```python
from build123d import *

# Parameters (mm, degrees)
BOSS_EXTRUDE1_DEPTH = 1.5875
CUT_EXTRUDE1_DEPTH  = 288.311537501
CUT_EXTRUDE2_DEPTH  = 1.5875
FILLET1_R           = 2.54


with BuildPart() as part:
    # Sketch2 → Boss-Extrude1 (new body)
    with BuildSketch(Plane(origin=(0, 0, 0), x_dir=(1, 0, 0), z_dir=(0, 1, 0))):
        Polygon((-122.047, 0), (0, 0), (122.047, 0), (11.684, -253.746), (6.35, -253.746), (6.35, -260.096), (-6.35, -260.096), (-6.35, -253.746), (-11.684, -253.746), align=None)
    extrude(amount=BOSS_EXTRUDE1_DEPTH)

    # Sketch3 → Cut-Extrude1 (cut, through all)
    with BuildSketch(Plane(origin=(0, 1.5875, 0), x_dir=(1, 0, 0), z_dir=(0, 1, 0))):
        Polygon((41.529, 0), (41.529, -4.7625), (119.975622372, -4.7625), (122.047, 0), align=None)
        Polygon((-119.975622372, -4.7625), (-122.047, 0), (-41.529, 0), (-41.529, -4.7625), align=None)
    extrude(amount=-CUT_EXTRUDE1_DEPTH, mode=Mode.SUBTRACT)

    # Sketch4 → Cut-Extrude2 (cut)
    with BuildSketch(Plane(origin=(0, 1.5875, 0), x_dir=(1, 0, 0), z_dir=(0, 1, 0))):
        Polygon((37.326544741, -116.821662879), (54.618110353, -116.821662879), (15.355253515, -207.09460645), align=None)
        Polygon((-34.444106562, -34.178727637), (41.755893438, -34.178727637), (0, -205.740215459), align=None)
        Polygon((58.747863162, -34.178727637), (90.562410016, -34.178727637), (59.474716621, -105.655380576), (41.351351035, -105.655380576), align=None)
        Polygon((-15.355253515, -207.09460645), (-37.326544741, -116.821662879), (-54.618110353, -116.821662879), align=None)
        Polygon((-41.351351035, -105.655380576), (-58.747863162, -34.178727637), (-90.562410016, -34.178727637), (-59.474716621, -105.655380576), align=None)
    extrude(amount=-CUT_EXTRUDE2_DEPTH, mode=Mode.SUBTRACT)

    # Fillet1
    fillet1_edges = [part.edges().sort_by_distance(p)[0] for p in [
        (-15.355253515, 0.79375, 207.09460645),
        (-54.618110353, 0.79375, 116.821662879),
        (-37.326544741, 0.79375, 116.821662879),
        (37.326544741, 0.79375, 116.821662879),
        (15.355253515, 0.79375, 207.09460645),
        (54.618110353, 0.79375, 116.821662879),
        (90.562410016, 0.79375, 34.178727637),
        (58.747863162, 0.79375, 34.178727637),
        (41.351351035, 0.79375, 105.655380576),
        (59.474716621, 0.79375, 105.655380576),
        (-41.351351035, 0.79375, 105.655380576),
        (-59.474716621, 0.79375, 105.655380576),
        (-90.562410016, 0.79375, 34.178727637),
        (-58.747863162, 0.79375, 34.178727637),
        (-34.444106562, 0.79375, 34.178727637),
        (0, 0.79375, 205.740215459),
        (41.755893438, 0.79375, 34.178727637),
    ]]
    fillet(fillet1_edges, radius=FILLET1_R)


solid = part.part
```
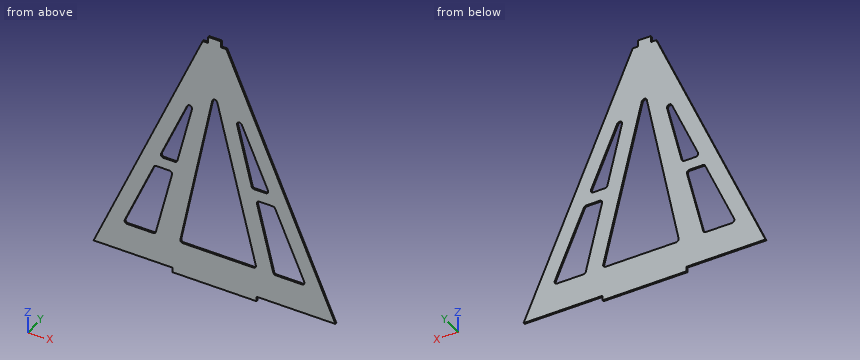
Here's how the part is built. I have some questions about the finished solid (model axes, mm). Coordinates: 2 decimals unless noted, no trailing zeros. Order: outer loops, then holes, each group sorted by start corner. A loop starts at its lowest first (then second) coordinate and runs counter-clockwise, first axis right, second up. Notation, with made-up numbers: (-6, 3) - (0, 3) arc R15 cw to (0, 10) - close; hole circle Ø4 at (-16, 87). An arc over 180 degrees is marked (long way). One line per question, with ' | ' between items. Start each with the question number.
1. If we section it at B-B (z = 111): Write out the boundary of the cut face in (x, y), and give its area (3 significant figures).
2. If we section it at D-D (y = 1.05): Give the number of separate pieces and of enclosed holes in the cut face, and give its area (3 significant figures).
3. If we section it at A-A (z = 65.5): Write out the boundary of the cut face in (x, y).
4. I'm going to push flat-ended pins straight in: pin 1 Ø0.5 at (x, y) = (97, 1) entering from -Z; pin 2 Ø0.8 at (x, y) = (9.5, 1) entering from +Z; pin 3 Ø0.8 at (x, y) = (43, 1) entering from +Z. Where does each tip first touch, or does it pass through?
5. If we section it at C-C (x = -72): Write out the boundary of the cut face in (y, z).
6. Please list where these lines run through material, in increasing order: line 1 along X through (y, z) = (0.6, 68); line 2 along X through (y, z) = (0.4, 173); line 3 along Z through (x, y) = (-66, 0.8). Write a range as [from, to].
Model answer:
1) outline: (-73.77, 0) - (-19.02, 0) - (-19.02, 1.59) - (-73.77, 1.59) - close; (23.06, 0) - (73.77, 0) - (73.77, 1.59) - (23.06, 1.59) - close | area: 167 mm²
2) separate pieces: 1 | enclosed holes: 5 | area: 21,800 mm²
3) outline: (-93.56, 0) - (-76.94, 0) - (-76.94, 1.59) - (-93.56, 1.59) - close; (-51.12, 0) - (-28.16, 0) - (-28.16, 1.59) - (-51.12, 1.59) - close; (34.13, 0) - (51.12, 0) - (51.12, 1.59) - (34.13, 1.59) - close; (76.94, 0) - (93.56, 0) - (93.56, 1.59) - (76.94, 1.59) - close
4) pin 1: stops at z = 4.76 | pin 2: stops at z = 253.75 | pin 3: stops at z = 182.66
5) outline: (0, 4.76) - (1.59, 4.76) - (1.59, 34.18) - (0, 34.18) - close; (0, 76.86) - (1.59, 76.86) - (1.59, 115.07) - (0, 115.07) - close
6) line 1: x = [-92.47, -75.85], [-50.52, -27.65], [33.52, 50.52], [75.85, 92.47] | line 2: x = [-46.8, -30.18], [-23.65, -6.57], [7.97, 23.65], [30.18, 46.8] | line 3: z = [4.76, 34.18], [90.65, 128.86]
